Geometry: final body of the model. Coordinates: model frame, mm. A direction names the side the tool comes from. Round coordinates to 2 decimals unless told otherwise and drop trailing zeros. Write each loop counter-clockwise with the first axis right and the second up, starting at its lowest first coordinate (ties: lowest second). Pieces come first, ordered by that corner, then holes. Notation, with made-up numbers: (83.5, -10.5) - (122.5, -10.5) arc R24 cw to (122.5, 16.5) - close; hole circle Ø4 at (-19, -25). An arc over 180 degrees is marked (long way). Use a Markdown table: item, result. Add a question column.
```python
from build123d import *

# Parameters (mm, degrees)
BOSS_EXTRUDE1_DEPTH      = 77.5
BOSS_EXTRUDE1_DEPTH_BACK = 77.5
SKETCH2_R                = 52.5
BOSS_EXTRUDE2_DEPTH      = 20
SKETCH3_W                = 135
SKETCH3_H                = 30
CUT_EXTRUDE1_DEPTH       = 135.768319719
HOLE1_D                  = 12
HOLE1_DEPTH              = 20
CIRPATTERN1_COUNT        = 6


with BuildPart() as part:
    # Sketch1 → Boss-Extrude1 (new, two sides: drawn at the far end of the back side and taken through both)
    with BuildSketch(Plane(origin=(0, 0, 0), x_dir=(0, 0, -1), z_dir=(1, 0, 0)).offset(-BOSS_EXTRUDE1_DEPTH_BACK)):
        Polygon((0, 40), (60, 40), (60, -40), (0, -40), (0, -30), (50, -30), (50, 30), (0, 30), align=None)
    extrude(amount=BOSS_EXTRUDE1_DEPTH + BOSS_EXTRUDE1_DEPTH_BACK)

    # Sketch2 → Boss-Extrude2 (add)
    with BuildSketch(Plane.XY):
        Circle(SKETCH2_R)
    extrude(amount=-BOSS_EXTRUDE2_DEPTH)

    # Sketch3 → Cut-Extrude1 (cut, through all)
    with BuildSketch(Plane(origin=(0, 40, 0), x_dir=(1, 0, 0), z_dir=(0, 1, 0))):
        with Locations((0, 35)):
            Rectangle(SKETCH3_W, SKETCH3_H)
    extrude(amount=-CUT_EXTRUDE1_DEPTH, mode=Mode.SUBTRACT)

    # Hole1
    with Locations(Plane.XY):
        with Locations((35, 0)):
            hole1 = Hole(HOLE1_D / 2, depth=HOLE1_DEPTH)

    # CirPattern1: Hole1 ×6 about axis
    cirpattern1_axis = Axis((-0.392370816, 0, 0), (0, 0, 1))
    for i in range(1, CIRPATTERN1_COUNT):
        add(hole1.rotate(cirpattern1_axis, i * 360 / CIRPATTERN1_COUNT), mode=Mode.SUBTRACT)


solid = part.part
```
1) Material intervals for L1, parallel to Y at x = -56.5, z = -7.5; L2, parallel to X at y = -39, z = -41; L3, parallel to Y at x = 43.5, z = -2.5, sorted ascending. Write a range as from..to.
2) Section A-A, the plane y = 0. Return the cut outline in (x, z).
3) Set-up query: faces 5 (the flat face through (-1, 1, -20)), 6 (the cylindrical face through (23.027, -32.453, -10.14)), 7 (the flat face through (63.9, 30, -19.8)), 8 (the flat face through (-64.4, 30, -19.8)). Return all of +Z, -Z, +X, -X, +Y, -Y with unobstructed straight access to the full face (end or side cutting, diameter ignored); none if empty.
4) Draft query along Z for faces 1 (the flat face through (-67.5, -35, -35)), 2 (the flat face through (-1, 1, 0)), 3 (the flat face through (-1, 40, -56)), 4 (the flat face through (67.5, 35, -35)). Return one class per face: released by +Z, released by -Z, zero draft, split by the parting line, or undercut.
5) Section B-B, the plane z = -39.5. Return the cut outline in (x, y).
6) Section C-C, the plane y = 14. Return the cut outline in (x, z), then the cut area to 3 significant figures.
7) Pin query (flat end, axial travel): P1, Ø17, axis at x = 57.5, z = -17.5, coming from the -Y side; P2, Ø6, axis at x = -25.5, z = -12.5, coming from the -Y side; P3, Ø12, axis at x = 36.5, z = -19.5, coming from the -Y side. Return the tip coordinate at first contact, or that it passes through.
8) Section D-D, the plane z = -54.5. Return the cut outline in (x, y), then the cut area to 3 significant figures.
Output values:
| question | item | result |
|---|---|---|
| 1 | L1 | y = -40..-30, 30..40 |
| 1 | L2 | x = -77.5..-67.5, 67.5..77.5 |
| 1 | L3 | y = -40..-30, -29.39..29.39, 30..40 |
| 2 | outline | (-77.5, -60) - (77.5, -60) - (77.5, -50) - (-77.5, -50) - close; (-52.5, -20) - (-41.78, -20) - (-41.78, 0) - (-52.5, 0) - close; (-29.78, -20) - (29, -20) - (29, 0) - (-29.78, 0) - close; (41, -20) - (52.5, -20) - (52.5, 0) - (41, 0) - close |
| 3 | face 5 | +Y, -Y |
| 3 | face 6 | +Z |
| 3 | face 7 | +Z, +X |
| 3 | face 8 | +Z, -X |
| 4 | face 1 | undercut |
| 4 | face 2 | released by +Z |
| 4 | face 3 | zero draft |
| 4 | face 4 | undercut |
| 5 | outline | (-77.5, -40) - (-67.5, -40) - (-67.5, -30) - (-77.5, -30) - close; (-77.5, 30) - (-67.5, 30) - (-67.5, 40) - (-77.5, 40) - close; (67.5, -40) - (77.5, -40) - (77.5, -30) - (67.5, -30) - close; (67.5, 30) - (77.5, 30) - (77.5, 40) - (67.5, 40) - close |
| 6 | outline | (-77.5, -60) - (77.5, -60) - (77.5, -50) - (-77.5, -50) - close; (-50.6, -20) - (50.6, -20) - (50.6, 0) - (-50.6, 0) - close |
| 6 | area | 3,570 mm^2 |
| 7 | P1 | stops at y = -40 |
| 7 | P2 | stops at y = -47.43 |
| 7 | P3 | stops at y = -42.73 |
| 8 | outline | (-77.5, -40) - (77.5, -40) - (77.5, 40) - (-77.5, 40) - close |
| 8 | area | 12,400 mm^2 |
